Source: CAD feature listing. Evaluate the final solid. Frame: model axes, mm. Give positions to 0.01 mm unless a question says otherwise; leave off trailing zeros. Order: outer loops, then holes, each group sorted by start corner. A loop starts at its lowest first (then second) coordinate and runs counter-clockwise, first axis right, second up.
```python
from build123d import *

# Parameters (mm, degrees)
CROQUIS2_W              = 80
CROQUIS2_H              = 80
SALIENTE_EXTRUIR1_DEPTH = 20
REDONDEO1_R             = 10
REDONDEO2_R             = 10
CROQUIS3_R              = 10
CORTAR_EXTRUIR1_DEPTH   = 79.988983231


with BuildPart() as part:
    # Croquis2 → Saliente-Extruir1 (new body)
    with BuildSketch(Plane(origin=(0, 0, 0), x_dir=(1, 0, 0), z_dir=(0, 1, 0))):
        with Locations((-24.623955432, -0.77994429)):
            Rectangle(CROQUIS2_W, CROQUIS2_H)
    extrude(amount=SALIENTE_EXTRUIR1_DEPTH)

    # Redondeo1
    redondeo1_edges = [part.edges().sort_by_distance(p)[0] for p in [
        (15.376044568, 10, 40.77994429),
    ]]
    fillet(redondeo1_edges, radius=REDONDEO1_R)

    # Redondeo2
    redondeo2_edges = [part.edges().sort_by_distance(p)[0] for p in [
        (-64.623955432, 10, 40.77994429),
    ]]
    fillet(redondeo2_edges, radius=REDONDEO2_R)

    # Croquis3 → Cortar-Extruir1 (cut, through all)
    with BuildSketch(Plane(origin=(0, 20, 0), x_dir=(1, 0, 0), z_dir=(0, 1, 0))):
        with Locations(Location((-46.623955432, -10.77994429, 0), (0, 0, 270))):
            Circle(CROQUIS3_R)
        with Locations(Location((-2.623955432, -10.77994429, 0), (0, 0, 90))):
            Circle(CROQUIS3_R)
    extrude(amount=-CORTAR_EXTRUIR1_DEPTH, mode=Mode.SUBTRACT)


solid = part.part
```
1) Draft query along X for faces 1 (the cylindrical face through (12.4, 10.1, 37.9)), 2 (the cylindrical face through (-56.386, 10.14, 8.612)), 3 (the flat face through (-64.624, 10, -4)). Return one class per face: +X half, -X half, draft (parallel to the pull), parting line (faces both ways), or undercut.
Report:
face 1: +X half
face 2: undercut
face 3: -X half
2) Section query C-C, the plane y = 13.25. Return the cut outline in (x, z), and give its area (3 significant figures).
Report:
outline: (-64.62, -39.22) - (15.38, -39.22) - (15.38, 30.78) arc R10 ccw to (5.38, 40.78) - (-54.62, 40.78) arc R10 ccw to (-64.62, 30.78) - close; hole circle Ø20 at (-46.62, 10.78); hole circle Ø20 at (-2.62, 10.78)
area: 5,730 mm2
3) Material intervals for L1, parallel to X at y = 12.25, z = 19.5; L2, parallel to X at y = 16.5, z = 14; L3, parallel to Z at x = -38, y = 13.5, sorted ascending.
Report:
L1: x = -64.62 to -51.52, -41.73 to -7.52, 2.27 to 15.38
L2: x = -64.62 to -56.09, -37.16 to -12.09, 6.84 to 15.38
L3: z = -39.22 to 5.72, 15.84 to 40.78
4) Section query D-D, the plane x = -50. Return the cut outline in (y, z), and give its area (3 significant figures).
Report:
outline: (0, -39.22) - (20, -39.22) - (20, 1.37) - (0, 1.37) - close; (0, 20.19) - (20, 20.19) - (20, 40.78) - (0, 40.78) - close
area: 1,220 mm2
5) Section query A-A, the plane x = -41. Return the cut outline in (y, z), and give its area (3 significant figures).
Report:
outline: (0, -39.22) - (20, -39.22) - (20, 2.51) - (0, 2.51) - close; (0, 19.05) - (20, 19.05) - (20, 40.78) - (0, 40.78) - close
area: 1,270 mm2
6) Section query B-B, the plane z = 19. Return the cut outline in (x, y), and give its area (3 significant figures).
Report:
outline: (-64.62, 0) - (-52.32, 0) - (-52.32, 20) - (-64.62, 20) - close; (-40.93, 0) - (-8.32, 0) - (-8.32, 20) - (-40.93, 20) - close; (3.07, 0) - (15.38, 0) - (15.38, 20) - (3.07, 20) - close
area: 1,140 mm2
